Geometry check sheet. Reference: drawing and pictorial views, mm from the part's lowest x, y, z. Give positions to 0.01 mm unless a question says otherwise; leave off trailing zeros. Write each loop counter-clockwise with the first axis right and the second up, starting at its lowest first coordinate (ties: lowest second). Pieces come first, ordered by that corner, then holes. Notation, with made-up numbers: M -29.5,-14.75 L 17.5,-14.75 A11 cw 17.5,6.25 Z; hole C 69.25,64.25 d9. An arc over 180 degrees is marked long. Answer as a JSON object with one key per item and string values.
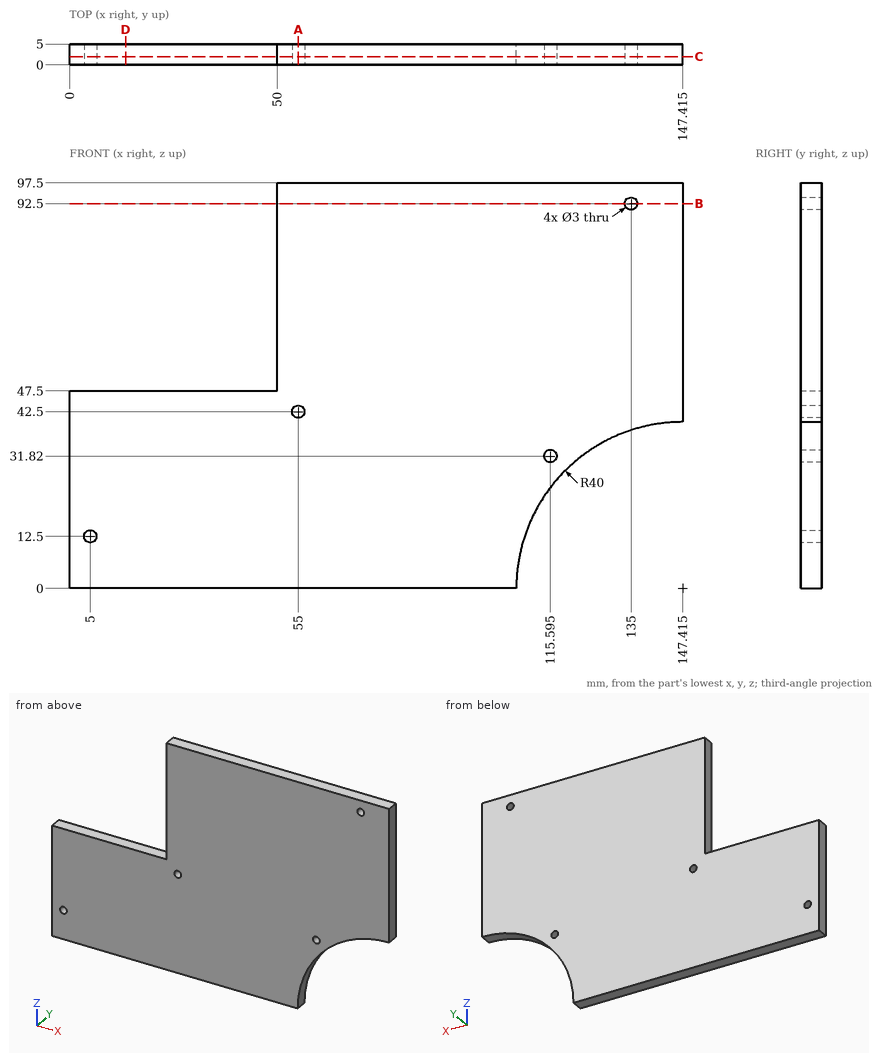
1) Section check A-A on x = 55. Record the boundary of the cut face in (y, z).
Completed:
{"outline": "M 0,0 L 5,0 L 5,41 L 0,41 Z; M 0,44 L 5,44 L 5,97.5 L 0,97.5 Z"}
2) Section check B-B on z = 92.5. Record the boundary of the cut face in (x, y) (3 decimals), and give its area (3 significant figures).
Completed:
{"outline": "M 50,0 L 133.5,0 L 133.5,5 L 50,5 Z; M 136.5,0 L 147.415,0 L 147.415,5 L 136.5,5 Z", "area": "472 mm2"}
3) Section check C-C on y = 1.95. Record the boundary of the cut face in (x, z) (1 decimal).
Completed:
{"outline": "M 0,0 L 107.4,0 A40 cw 147.4,40 L 147.4,97.5 L 50,97.5 L 50,47.5 L 0,47.5 Z; hole C 5,12.5 d3; hole C 55,42.5 d3; hole C 115.6,31.8 d3; hole C 135,92.5 d3"}
4) Thickness scan on L1, parallel to Z at x = 55, y = 1.5; L2, parallel to X at y = 2.8, z = 42.5 (3 decimals); L3, parallel to Z at x = 39.5, y = 1.75. Record the ranges inside material, lowest first.
Completed:
{"L1": "z = 0 to 41, 44 to 97.5", "L2": "x = 0 to 53.5, 56.5 to 147.415", "L3": "z = 0 to 47.5"}
5) Section check D-D on x = 13.5. Record the boundary of the cut face in (y, z).
Completed:
{"outline": "M 0,0 L 5,0 L 5,47.5 L 0,47.5 Z"}
